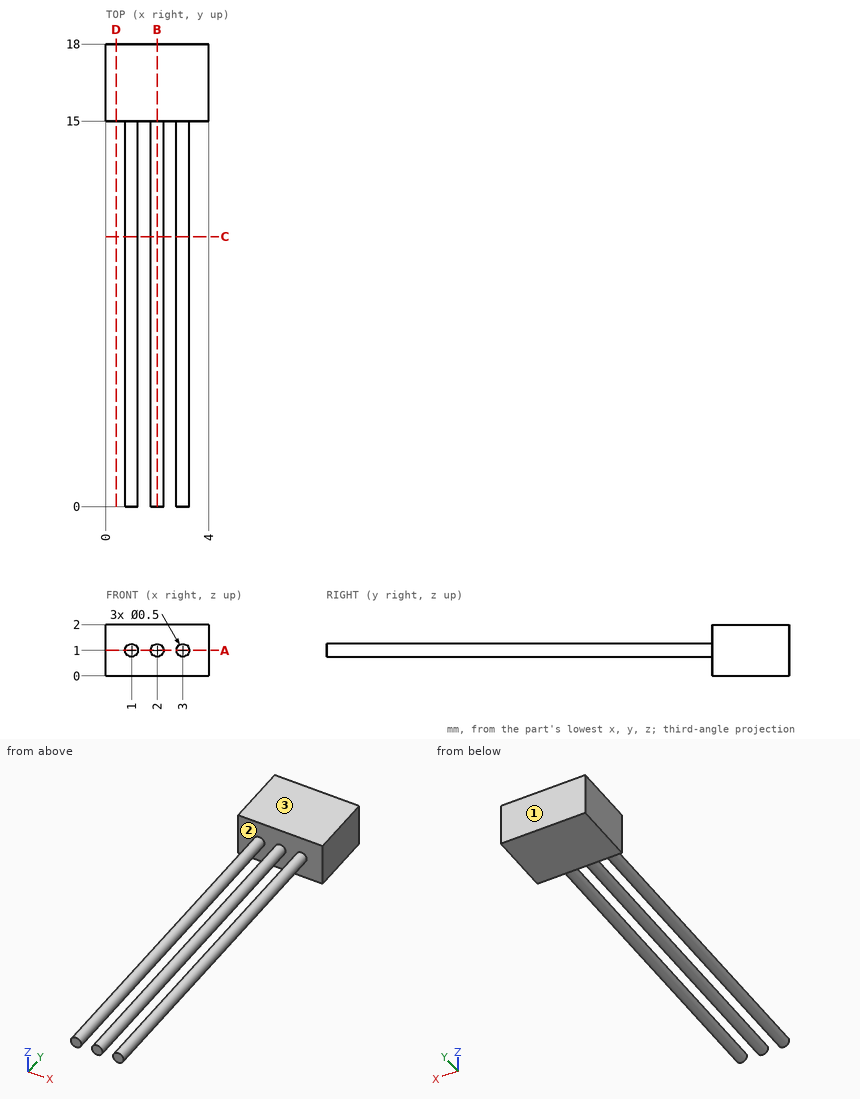
Input: dimensioned drawing with shaded views. Units: mm. Origin: part minimum x, y, z. Round coordinates to 2 decimals unless told otherwise and drop trailing zeros. Loops run counter-clockwise (first coordinate to the right, second up) from the corner with the lowest first, then second, coordinate; pieces in that order, holes last.
1) Section query D-D on x = 0.4. Return the cut outline in (y, z), plus the area to 3 significant figures.
Ans:
outline: (15, 0) - (18, 0) - (18, 2) - (15, 2) - close
area: 6.00 mm2
2) Section query C-C on y = 10.5. Return the cut outline in (x, z), plus the area to 3 significant figures.
Ans:
outline: circle Ø0.5 at (1, 1); circle Ø0.5 at (2, 1); circle Ø0.5 at (3, 1)
area: 0.589 mm2
3) Pin query (flat end, axial travel): pin 1 (2 mm diameter, centred on x = 1.5, y = 12.5, fed in from +Z); pin 2 (1.5 mm diameter, centred on x = 0.5, y = 8.5, fed in from -Z). Return the tip coordinate at first contact, or that it passes through.
Ans:
pin 1: stops at z = 1.25
pin 2: stops at z = 0.75
4) Section query B-B on x = 2. Return the cut outline in (y, z).
Ans:
outline: (0, 0.75) - (15, 0.75) - (15, 0) - (18, 0) - (18, 2) - (15, 2) - (15, 1.25) - (0, 1.25) - close
5) Pull-direction query (Y, two-part tool) for the marked faces 1, 2 and 3; classes: released by +Y, released by -Y, zero draft, split by the parting line, or undercut.
Ans:
face 1: released by +Y
face 2: released by -Y
face 3: zero draft
6) Material intervals for line 1 (X direction, y = 1.25, z = 0.95); line 2 (Y direction, x = 0.55, z = 1.55); line 3 (X direction, y = 9.25, z = 1.2), sorted ascending.
Ans:
line 1: x = 0.76 to 1.24, 1.76 to 2.24, 2.76 to 3.24
line 2: y = 15 to 18
line 3: x = 0.85 to 1.15, 1.85 to 2.15, 2.85 to 3.15
7) Section query A-A on z = 1. Return the cut outline in (x, y).
Ans:
outline: (0, 15) - (0.75, 15) - (0.75, 0) - (1.25, 0) - (1.25, 15) - (1.75, 15) - (1.75, 0) - (2.25, 0) - (2.25, 15) - (2.75, 15) - (2.75, 0) - (3.25, 0) - (3.25, 15) - (4, 15) - (4, 18) - (0, 18) - close
